Drawing for the job (mm, zero at the part's lowest x, y, z). A direction names the side the tool comes from. Coordinates: 2 decimals unless noted, no trailing zeros. Loops run counter-clockwise (first coordinate to the right, second up) from the corner with the lowest first, then second, coordinate; pieces in that order, holes last. Notation, with made-up numbers: (-26.5, 28) - (-2.5, 28) arc R27 cw to (-2.5, 66) - close; hole circle Ø8 at (4.25, 78.25). An arc over 180 degrees is marked (long way). Put each result on its own line as item: value.
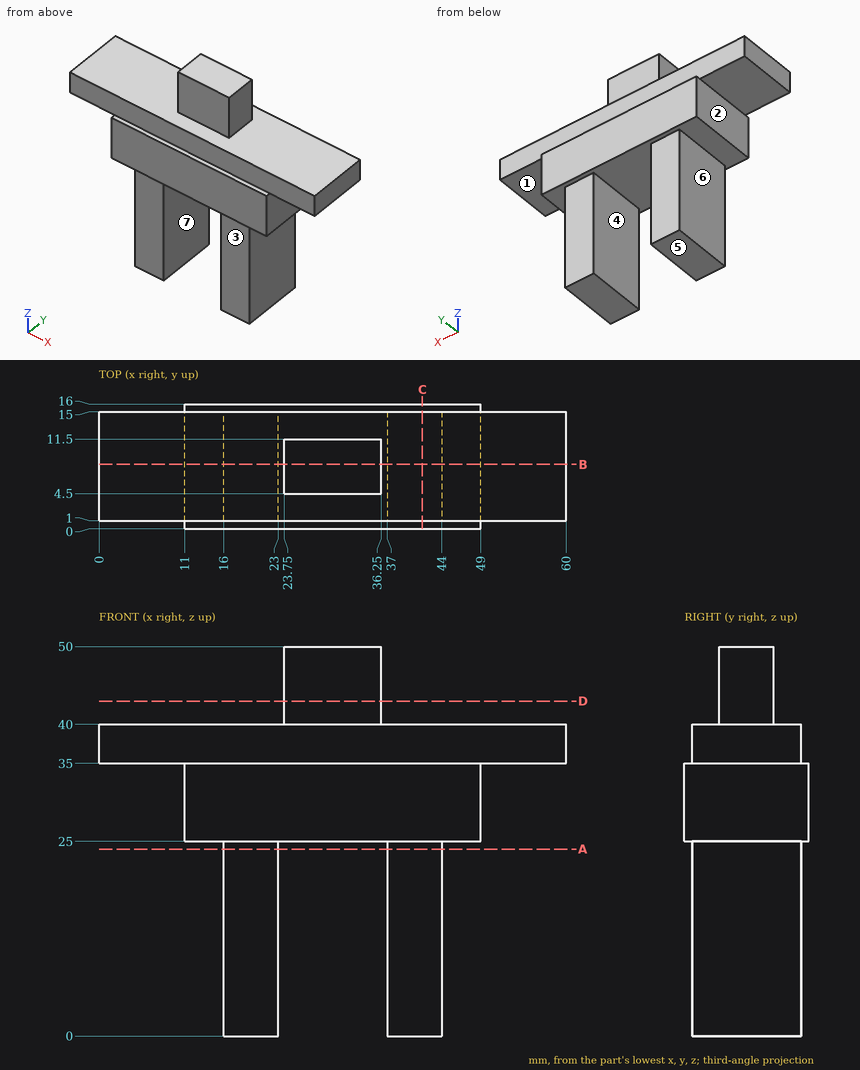
Q1. Wall check: L1, parallel to X at y = 7.5, z = 9.5; L2, parallel to Z at x = 10, y = 6; L3, parallel to X at y = 14.5, z = 30.5. Give the ranges that are in metal, low to high. Write a range as from..to.
Determined:
L1: 16..23, 37..44
L2: 35..40
L3: 11..49
Q2. Pin check, flat tips, straight feed: pin 1 Ø4 at (y, z) = (6, 13.5) entering from -X; pin 2 Ø11 at (x, z) = (27, 42.5) entering from -Y; pin 3 Ø3 at (y, z) = (9, 28) entering from -X. Stop position of each tip, or through.
Determined:
pin 1: x = 16
pin 2: y = 1
pin 3: x = 11
Q3. Slice it at A-A, the plane z = 24. Give the cut face in (x, y).
Determined:
outline: (16, 1) - (23, 1) - (23, 15) - (16, 15) - close; (37, 1) - (44, 1) - (44, 15) - (37, 15) - close
Q4. Mould opens along X. For the marked faces 4, 5, 6 and 7 say: +X half, -X half, draft (parallel to the pull), parting line (faces both ways), or undercut.
Determined:
face 4: undercut
face 5: draft
face 6: -X half
face 7: undercut
Q5. Slice it at C-C, the plane x = 41.5. Give the cut face in (y, z), then the cut area to 3 significant figures.
Determined:
outline: (0, 25) - (1, 25) - (1, 0) - (15, 0) - (15, 25) - (16, 25) - (16, 35) - (15, 35) - (15, 40) - (1, 40) - (1, 35) - (0, 35) - close
area: 580 mm2
Q6. Tool access for the marked faces 1, 2 and 3: list every direction of +Z, -Z, +X, -X, +Y, -Y with a clear straight run to the whole face (end or side of a thin tool).
Determined:
face 1: -Z, +X, +Y, -Y
face 2: -Z, -X, +Y, -Y
face 3: -Z, +X, -X, -Y
Q7. Slice it at B-B, the plane y = 8.25. Give the cut face in (x, z), then the cut area to 4 significant figures.
Determined:
outline: (0, 35) - (11, 35) - (11, 25) - (16, 25) - (16, 0) - (23, 0) - (23, 25) - (37, 25) - (37, 0) - (44, 0) - (44, 25) - (49, 25) - (49, 35) - (60, 35) - (60, 40) - (36.25, 40) - (36.25, 50) - (23.75, 50) - (23.75, 40) - (0, 40) - close
area: 1,155 mm2
Q8. Slice it at D-D, the plane z = 43. Give the cut face in (x, y).
Determined:
outline: (23.75, 4.5) - (36.25, 4.5) - (36.25, 11.5) - (23.75, 11.5) - close
